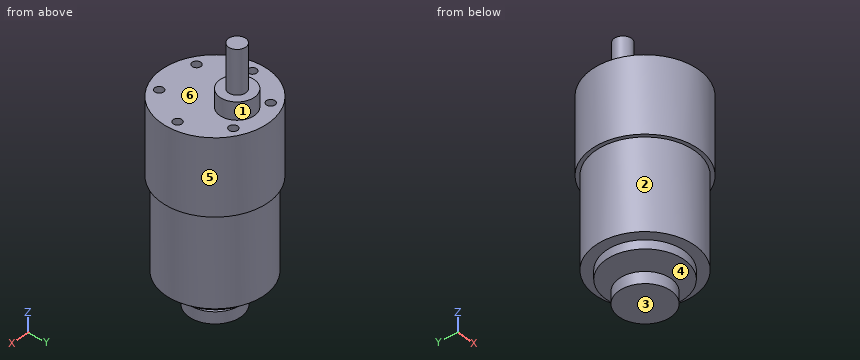
```python
from build123d import *

# Parameters (mm, degrees)
ESQUISSE1_R             = 18.5
BOSS_EXTRU_1_DEPTH      = 26
ESQUISSE2_R             = 17.2
BOSS_EXTRU_2_DEPTH      = 31
ESQUISSE3_R             = 13.55
BOSS_EXTRU_3_DEPTH      = 3
ESQUISSE4_R             = 0.75
BOSS_EXTRU_4_DEPTH      = 4
ESQUISSE5_R             = 9
BOSS_EXTRU_5_DEPTH      = 4
ESQUISSE6_R             = 6
BOSS_EXTRU_7_DEPTH      = 6
ESQUISSE8_R             = 3
BOSS_EXTRU_8_DEPTH      = 15
ESQUISSE9_R             = 1.5
ENL_V_MAT_EXTRU_4_DEPTH = 5


with BuildPart() as part:
    # Esquisse1 → Boss.-Extru.1 (new body)
    with BuildSketch(Plane.XY):
        with Locations(Location((0, 0, 0), (0, 0, 180))):
            Circle(ESQUISSE1_R)
    extrude(amount=BOSS_EXTRU_1_DEPTH)

    # Esquisse2 → Boss.-Extru.2 (add)
    with BuildSketch(Plane(origin=(0, 0, 0), x_dir=(-1, 0, 0), z_dir=(0, 0, -1))):
        with Locations(Location((0, 0, 0), (0, 0, 180))):
            Circle(ESQUISSE2_R)
    extrude(amount=BOSS_EXTRU_2_DEPTH)

    # Esquisse3 → Boss.-Extru.3 (add)
    with BuildSketch(Plane(origin=(0, 0, -31), x_dir=(-1, 0, 0), z_dir=(0, 0, -1))):
        Circle(ESQUISSE3_R)
    extrude(amount=BOSS_EXTRU_3_DEPTH)

    # Esquisse4 → Boss.-Extru.4 (add)
    with BuildSketch(Plane(origin=(0, 0, -34), x_dir=(-1, 0, 0), z_dir=(0, 0, -1))):
        Circle(ESQUISSE4_R)
    extrude(amount=BOSS_EXTRU_4_DEPTH)

    # Esquisse5 → Boss.-Extru.5 (add)
    with BuildSketch(Plane(origin=(0, 0, -38), x_dir=(-1, 0, 0), z_dir=(0, 0, -1))):
        Circle(ESQUISSE5_R)
    extrude(amount=BOSS_EXTRU_5_DEPTH)

    # Esquisse6 → Boss.-Extru.7 (add)
    with BuildSketch(Plane.XY.offset(26)):
        with Locations((-0.326961586, 7.492869685)):
            Circle(ESQUISSE6_R)
    extrude(amount=BOSS_EXTRU_7_DEPTH)

    # Esquisse8 → Boss.-Extru.8 (add)
    with BuildSketch(Plane.XY.offset(32)):
        with Locations((-0.326961586, 7.492869685)):
            Circle(ESQUISSE8_R)
    extrude(amount=BOSS_EXTRU_8_DEPTH)

    # Esquisse9 → Enlèv. mat.-Extru.4 (cut)
    with BuildSketch(Plane.XY.offset(26)):
        with Locations((15, 0)):
            Circle(ESQUISSE9_R)
        with Locations((7.5, -12.990381057)):
            Circle(ESQUISSE9_R)
        with Locations((-7.5, -12.990381057)):
            Circle(ESQUISSE9_R)
        with Locations((-15, 0)):
            Circle(ESQUISSE9_R)
        with Locations((-7.5, 12.990381057)):
            Circle(ESQUISSE9_R)
        with Locations((7.5, 12.990381057)):
            Circle(ESQUISSE9_R)
    extrude(amount=-ENL_V_MAT_EXTRU_4_DEPTH, mode=Mode.SUBTRACT)


solid = part.part
```
CAD build for the part. Positions are in the model's coordinates, mm. Face numbers are marked on the shaded views. A direction names the side the tool comes from. Give positions to 0.01 mm unless a question says otherwise; leave off trailing zeros. Write each loop counter-clockwise with the first axis right and the second up, starting at its lowest first coordinate (ties: lowest second). Pieces come first, ordered by that corner, then holes. Notation, with made-up numbers: M 71,89 L 75,89 A14 cw 75,95 Z; hole C 80,13.5 d4. An arc over 180 degrees is marked long. Return JSON: item names as keys, results as strings. Group by question number.
(1) Band-saw the part on A-A (x = -7.5). Give the cut face in (y, z), and give its area (3 significant figures).
(2) Band-saw the part on D-D (x = 15). Give the cut face in (y, z).
(3) Drill centre lines: L1, parallel to Y at x = 7.5, z = 23.9; L2, parallel to Z at x = -6, y = 3.5; L3, parallel to Z at x = 16, y = 4.5. Where is each one in solid material? Low to high. Write a range as [from, to].
(4) Mould opens along Z. For the marked faces 3, 4, 5 and 6 say: pulls with the +Z half, pulls with the -Z half, needs draft (parallel to the pull), parting line crosses it, or undercut.
(5) Flat gauge pins, fed straight in: pin 1 Ø2.5 at (x, y) = (-7.5, -12.99) entering from -Z; pin 2 Ø3.5 at (x, y) = (7.5, 12.5) entering from +Z; pin 3 Ø6 at (x, z) = (3, 8) entering from -Y. Where does each tip first touch, or does it go through?
(6) 3-axis set-ups, long thin cutter, end or side, ignore diameter. For the marked faces 1 and 2: which of +Z, -Z, +X, -X, +Y, -Y reach the whole face in a straight line?
(7) Band-saw the part on C-C (z = 11). Give the cut face in (x, y).
(8) Band-saw the part on B-B (y = -7.5). Give the cut face in (x, z), and give its area (3 significant figures).
Entries:
{
 "1": {"outline": "M -16.91,0 L -15.48,0 L -15.48,-31 L -11.29,-31 L -11.29,-34 L 11.29,-34 L 11.29,-31 L 15.48,-31 L 15.48,0 L 16.91,0 L 16.91,26 L 14.49,26 L 14.49,21 L 11.49,21 L 11.49,26 L -11.49,26 L -11.49,21 L -14.49,21 L -14.49,26 L -16.91,26 Z; M -4.97,-42 L 4.97,-42 L 4.97,-38 L -4.97,-38 Z", "area": "1,920 mm^2"},
 "2": {"outline": "M -10.83,0 L -8.42,0 L -8.42,-31 L 8.42,-31 L 8.42,0 L 10.83,0 L 10.83,26 L 1.5,26 L 1.5,21 L -1.5,21 L -1.5,26 L -10.83,26 Z"},
 "3": {"L1": "y = [-16.91, -14.49], [-11.49, 11.49], [14.49, 16.91]", "L2": "z = [-42, -38], [-34, 26]", "L3": "z = [-31, 26]"},
 "4": {"face 3": "pulls with the -Z half", "face 4": "undercut", "face 5": "needs draft", "face 6": "pulls with the +Z half"},
 "5": {"pin 1": "stops at z = -31", "pin 2": "stops at z = 26", "pin 3": "stops at y = -18.5"},
 "6": {"face 1": "+Z", "face 2": "-Z"},
 "7": {"outline": "C 0,0 d37"},
 "8": {"outline": "M -16.91,0 L -15.48,0 L -15.48,-31 L -11.29,-31 L -11.29,-34 L 11.29,-34 L 11.29,-31 L 15.48,-31 L 15.48,0 L 16.91,0 L 16.91,26 L -16.91,26 Z; M -4.97,-42 L 4.97,-42 L 4.97,-38 L -4.97,-38 Z", "area": "1,950 mm^2"}
}
